CAD build for the part. Positions are in the model's coordinates, mm. Face numbers are marked on the shaded views. A direction names the side the tool comes from. Round coordinates to 2 decimals unless told otherwise and drop trailing zeros. Loops run counter-clockwise (first coordinate to the right, second up) from the corner with the lowest first, then second, coordinate; pieces in that order, holes last.
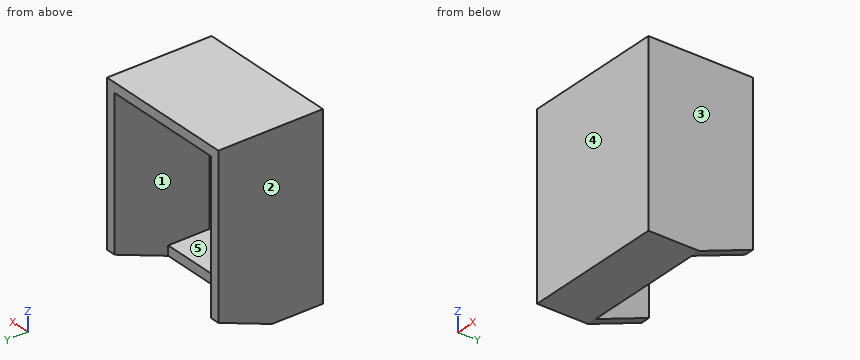
```python
from build123d import *

# Parameters (mm, degrees)
BOSS_EXTRUDE1_DEPTH = 104
SHELL1_T            = -7
SKETCH3_W           = 90
SKETCH3_H           = 18.2
CUT_EXTRUDE1_DEPTH  = 104


with BuildPart() as part:
    # Sketch1 → Boss-Extrude1 (new body)
    with BuildSketch(Plane(origin=(0, 0, 0), x_dir=(0, 0, -1), z_dir=(1, 0, 0))):
        Polygon((0, 0), (130, 0), (130, 37), (115, 76), (0, 76), align=None)
    extrude(amount=BOSS_EXTRUDE1_DEPTH)

    # Shell1
    shell1_openings = [part.faces().sort_by_distance(p)[0] for p in [
        (52, 76, -57.5),
        (52, 56.5, -122.5),
    ]]
    offset(amount=SHELL1_T, openings=shell1_openings, kind=Kind.INTERSECTION)

    # Sketch3 → Cut-Extrude1 (cut)
    with BuildSketch(Plane.XY.offset(-123)):
        with Locations((52, 46.1)):
            Rectangle(SKETCH3_W, SKETCH3_H)
    extrude(amount=-CUT_EXTRUDE1_DEPTH, mode=Mode.SUBTRACT)


solid = part.part
```
Item 1: Flat gauge pins, fed straight in: P1, Ø3.5, axis at x = 43.5, z = -126, coming from the +Y side; P2, Ø8, axis at x = 35, z = -91.5, coming from the +Y side; P3, Ø1, axis at x = 57, y = 63, coming from the -Z side. Where does each tip first touch, or does it go through?
Answers follow:
P1: stops at y = 37
P2: stops at y = 7
P3: stops at z = -7
Item 2: Cut at B-B, the plane y = 50. Give the cut face in (x, z).
Answers follow:
outline: (0, -125) - (7, -125) - (7, -7) - (97, -7) - (97, -125) - (104, -125) - (104, 0) - (0, 0) - close
Item 3: 3-axis set-ups, long thin cutter, end or side, ignore diameter. For the marked faces 4 and 5: which of +Z, -Z, +X, -X, +Y, -Y reach the whole face in a straight line?
Answers follow:
face 4: +Z, -Z, +X, -X, -Y
face 5: +Y
Item 4: Cut at C-C, the plane y = 15. Give the cut face in (x, z).
Answers follow:
outline: (0, -130) - (104, -130) - (104, 0) - (0, 0) - close; hole (7, -123) - (97, -123) - (97, -7) - (7, -7) - close
Item 5: Two-plate mould, pull along X, no slides. Class the marked faces 1, 2 and 3: released by +X, released by -X, zero draft, split by the parting line, or undercut.
Answers follow:
face 1: undercut
face 2: released by -X
face 3: released by +X
Item 6: Probe line 1 (Z direction, x = 57.5, y = 21.5); line 2 (X direction, y = 48, z = -77); line 3 (Y direction, x = 28, z = -64). List the from-to ranges inside material, lowest first.
Answers follow:
line 1: z = -130 to -123, -7 to 0
line 2: x = 0 to 7, 97 to 104
line 3: y = 0 to 7
Item 7: Cut at A-A, the plane z = -119.5. Give the cut face in (x, y), plus the area to 3 significant figures.
Answers follow:
outline: (0, 0) - (104, 0) - (104, 64.3) - (97, 64.3) - (97, 7) - (7, 7) - (7, 64.3) - (0, 64.3) - close
area: 1,530 mm2
